Job drawing, mm, ordinate dimensions from the low corner. One solid piece. A direction names the side the tool comes from. Round coordinates to 2 decimals unless told otherwise and drop trailing zeros. Loops run counter-clockwise (first coordinate to the right, second up) from the corner with the lowest first, then second, coordinate; pieces in that order, holes last.
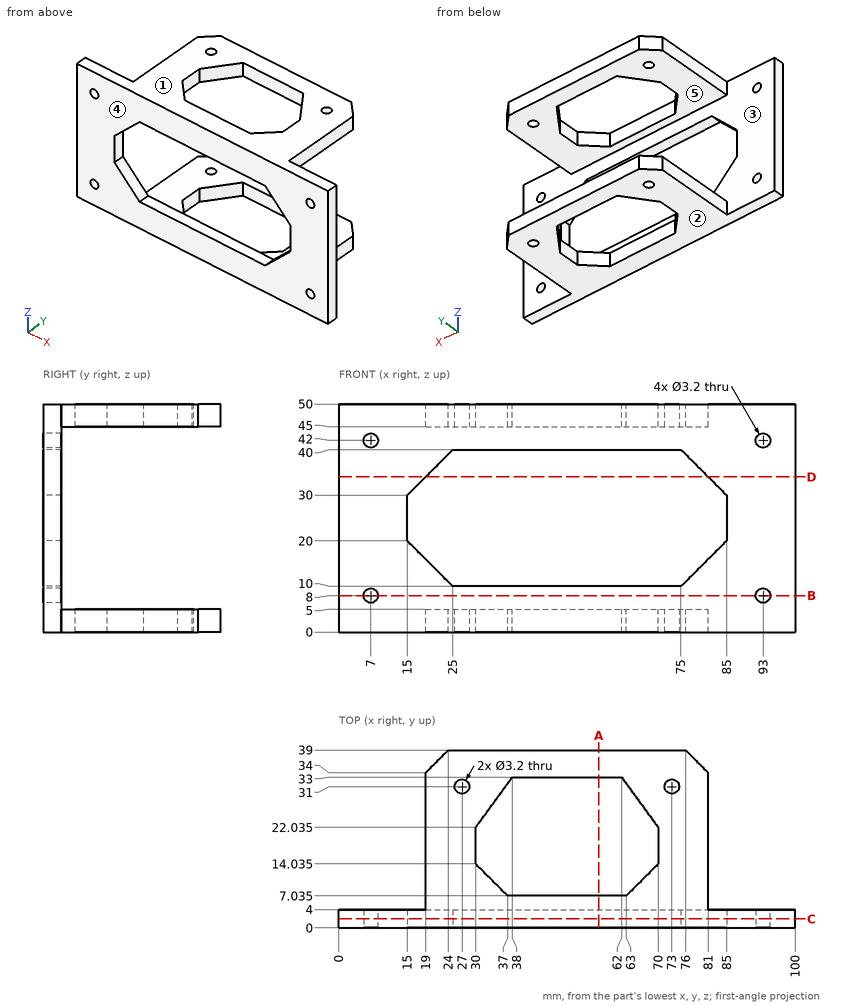
(1) Slice it at A-A on x = 57. List the corners of the cut face in (y, z) (1 decimal), plus the area to 3 significant figures.
Responses:
outline: (0, 0) - (7, 0) - (7, 5) - (4, 5) - (4, 10) - (0, 10) - close; (0, 40) - (4, 40) - (4, 45) - (7, 45) - (7, 50) - (0, 50) - close; (33, 0) - (39, 0) - (39, 5) - (33, 5) - close; (33, 45) - (39, 45) - (39, 50) - (33, 50) - close
area: 170 mm2
(2) Which spindle directions (+Z, -Z, +X, -X, +Y, -Y) get a long thin tool onto all of the face, cutting with end or side? Do the marked faces 4 and 5. Say none if no direction does.
Responses:
face 4: +Z, -Z, +X, -X, -Y
face 5: +X, -X, +Y
(3) Slice it at D-D on z = 34. List the corners of the cut face in (x, y), plus the area to 3 significant figures.
Responses:
outline: (0, 0) - (19, 0) - (19, 4) - (0, 4) - close; (81, 0) - (100, 0) - (100, 4) - (81, 4) - close
area: 152 mm2
(4) Pull direction Z, two halves, no side cores. Call the marked faces 1, 2 and 3: +Z half, -Z half, draft (parallel to the pull), parting line (faces both ways), or undercut.
Responses:
face 1: +Z half
face 2: -Z half
face 3: undercut
(5) Slice it at C-C on y = 2. List the corners of the cut face in (x, z), plus the area to 3 significant figures.
Responses:
outline: (0, 0) - (100, 0) - (100, 50) - (0, 50) - close; hole circle Ø3.2 at (7, 8); hole circle Ø3.2 at (7, 42); hole (15, 20) - (25, 10) - (75, 10) - (85, 20) - (85, 30) - (75, 40) - (25, 40) - (15, 30) - close; hole circle Ø3.2 at (93, 8); hole circle Ø3.2 at (93, 42)
area: 3,070 mm2
(6) Slice it at B-B on z = 8. List the corners of the cut face in (x, y).
Responses:
outline: (0, 0) - (5.4, 0) - (5.4, 4) - (0, 4) - close; (8.6, 0) - (91.4, 0) - (91.4, 4) - (8.6, 4) - close; (94.6, 0) - (100, 0) - (100, 4) - (94.6, 4) - close
(7) Pin check, flat tips, straight feed: P1, Ø1.5, axis at y = 19, z = 47, coming from the -X side; P2, Ø3.5, axis at x = 7, z = 8, coming from the +Y side; P3, Ø2.5, axis at y = 17.5, z = 2.5, coming from the +X side. Stop position of each tip, or through.
Responses:
P1: stops at x = 19
P2: stops at y = 4
P3: stops at x = 81
(8) Probe line 1 (Z direction, x = 93, y = 2.6); line 2 (Z direction, x = 33.5, y = 28); line 3 (Z direction, x = 26, y = 3.5). List the from-to ranges inside material, lowest first.
Responses:
line 1: z = 0 to 6.4, 9.6 to 40.4, 43.6 to 50
line 2: z = 0 to 5, 45 to 50
line 3: z = 0 to 10, 40 to 50
